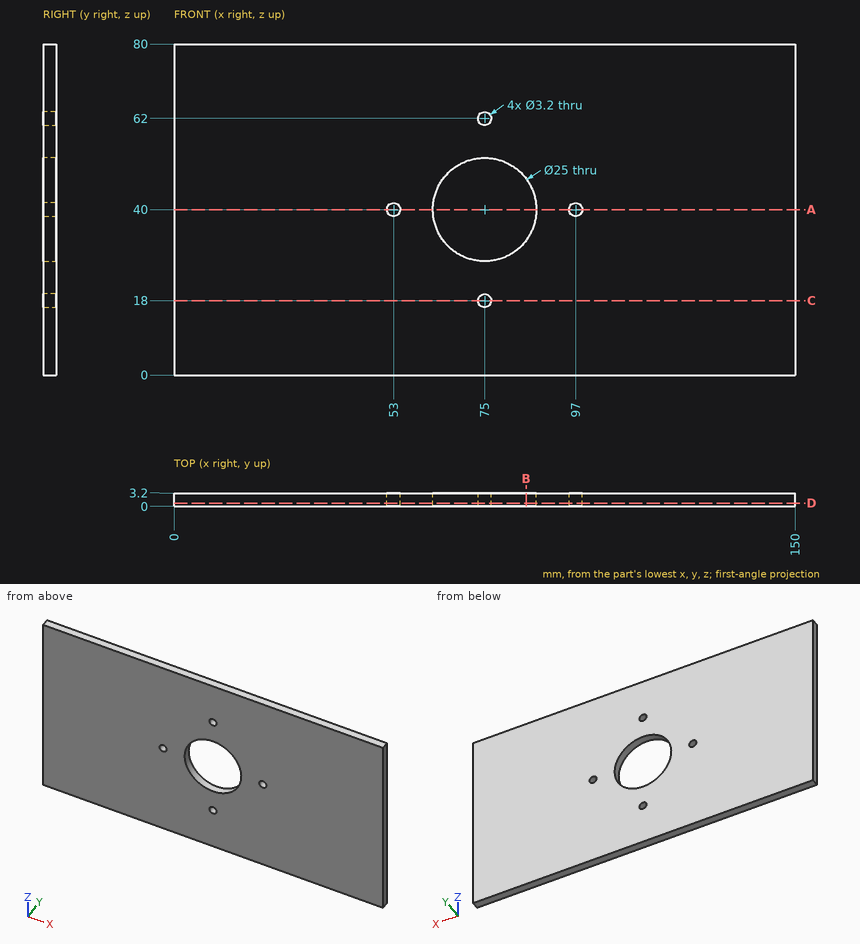
Study the drawing (mm; zero at the part's minimum x, y, z) and answer. Coordinates: 2 decimals unless noted, no trailing zeros. Write each loop counter-clockwise with the first axis right and the second up, starting at its lowest first coordinate (ties: lowest second). Pieces come first, ordered by that corner, then holes. Notation, with made-up numbers: M 47.25,69.25 L 87.25,69.25 A25 cw 87.25,107.25 Z; hole C 54.5,46.5 d11. An arc over 180 degrees is marked long. Use a Markdown table: item, result. Add a question column.
1. Straight lines are drawn through the part: line 1 along X through (y, z) = (1.4, 40); line 2 along X through (y, z) = (2.45, 62); line 3 along X through (y, z) = (2, 49.5). For each, find the intervals that lie inside material, in ascending order. Write a range as [from, to].
2. Section D-D (y = 0.75) is taken. Give the vertices of the cut face in (x, z), plus the area to 3 significant figures.
3. Given P1, Ø4, axis at x = 75, z = 18, coming from the +Y side, flat-ended and moving along its own axis, determine where the tip first touches the part or whether it passes through.
4. Section A-A (z = 40) is taken. Give the vertices of the cut face in (x, y), plus the area to 3 significant figures.
5. Section C-C (z = 18) is taken. Give the vertices of the cut face in (x, y), plus the area to 3 significant figures.
6. Section B-B (x = 85) is taken. Give the vertices of the cut face in (y, z), plus the area to 3 significant figures.
Data:
| question | item | result |
|---|---|---|
| 1 | line 1 | x = [0, 51.4], [54.6, 62.5], [87.5, 95.4], [98.6, 150] |
| 1 | line 2 | x = [0, 73.4], [76.6, 150] |
| 1 | line 3 | x = [0, 66.88], [83.12, 150] |
| 2 | outline | M 0,0 L 150,0 L 150,80 L 0,80 Z; hole C 53,40 d3.2; hole C 75,40 d25; hole C 75,18 d3.2; hole C 75,62 d3.2; hole C 97,40 d3.2 |
| 2 | area | 11,500 mm2 |
| 3 | P1 | stops at y = 3.2 |
| 4 | outline | M 0,0 L 51.4,0 L 51.4,3.2 L 0,3.2 Z; M 54.6,0 L 62.5,0 L 62.5,3.2 L 54.6,3.2 Z; M 87.5,0 L 95.4,0 L 95.4,3.2 L 87.5,3.2 Z; M 98.6,0 L 150,0 L 150,3.2 L 98.6,3.2 Z |
| 4 | area | 380 mm2 |
| 5 | outline | M 0,0 L 73.4,0 L 73.4,3.2 L 0,3.2 Z; M 76.6,0 L 150,0 L 150,3.2 L 76.6,3.2 Z |
| 5 | area | 470 mm2 |
| 6 | outline | M 0,0 L 3.2,0 L 3.2,32.5 L 0,32.5 Z; M 0,47.5 L 3.2,47.5 L 3.2,80 L 0,80 Z |
| 6 | area | 208 mm2 |
